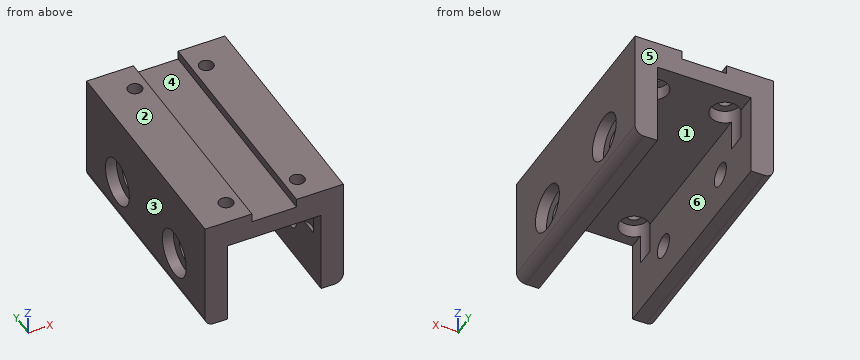
from build123d import *

# Parameters (mm, degrees)
PAD031_DEPTH            = 13.5
PAD031_DEPTH_BACK       = 38.5
SKETCH097_R             = 1.6
POCKET050_DEPTH         = 6.201
POCKET050_DEPTH_BACK    = 19.001
SKETCH100_R             = 3.25
POCKET051_DEPTH         = 10
LINEARPATTERN_COUNT     = 2
LINEARPATTERN_PITCH     = 25
BODY029_PLACEMENT_ANGLE = 180


with BuildPart() as part:
    # Sketch099 → Pad031 (new body, two sides)
    with BuildSketch(Plane.XZ) as pad031_sk:
        with BuildLine():
            Line((-13.5, 19), (-10.5, 19))
            Line((-10.5, 0), (-10.5, 19))
            Line((10.5, 0), (-10.5, 0))
            Line((10.5, 19), (10.5, 0))
            Line((10.5, 19), (13.5, 19))
            ThreePointArc((15.5, 17), (14.914214, 18.414214), (13.5, 19))
            Line((15.5, 17), (15.5, -6.2))
            Line((15.5, -6.2), (5, -6.2))
            Line((5, -4.2), (5, -6.2))
            Line((-5, -4.2), (5, -4.2))
            Line((-5, -6.2), (-5, -4.2))
            Line((-5, -6.2), (-15.5, -6.2))
            Line((-15.5, -6.2), (-15.5, 17))
            ThreePointArc((-13.5, 19), (-14.914214, 18.414214), (-15.5, 17))
        make_face()
    extrude(amount=PAD031_DEPTH)
    extrude(pad031_sk.sketch, amount=-PAD031_DEPTH_BACK)

    # Sketch097 → Pocket050 (cut, two sides)
    with BuildSketch(Plane.XY) as pocket050_sk:
        with Locations((-8, 32)):
            Circle(SKETCH097_R)
        with Locations((8, 32)):
            Circle(SKETCH097_R)
        with Locations((-8, -8)):
            Circle(SKETCH097_R)
        with Locations((8, -8)):
            Circle(SKETCH097_R)
    extrude(amount=-POCKET050_DEPTH, mode=Mode.SUBTRACT)
    extrude(pocket050_sk.sketch, amount=POCKET050_DEPTH_BACK, mode=Mode.SUBTRACT)

    # Sketch100 → Pocket051 (cut)
    with BuildSketch(Plane(origin=(0, 0, -3), x_dir=(-1, 0, 0), z_dir=(0, 0, -1))):
        with Locations((-8, 32)):
            Circle(SKETCH100_R)
        with Locations((8, 32)):
            Circle(SKETCH100_R)
        with Locations((-8, -8)):
            Circle(SKETCH100_R)
        with Locations((8, -8)):
            Circle(SKETCH100_R)
    extrude(amount=-POCKET051_DEPTH, mode=Mode.SUBTRACT)

    # Sketch110 → Groove (revolve, cut)
    with BuildSketch(Plane(origin=(0, 0, 10), x_dir=(-1, 0, 0), z_dir=(0, 1, 0))):
        Polygon((-13, 2.65), (13, 2.65), (13, 5.25), (23, 5.25), (23, 0), (-23, 0), (-23, 5.25), (-13, 5.25), align=None)
    groove = revolve(axis=Axis((0, 0, 10), (-1, 0, 0)), mode=Mode.SUBTRACT)

    # LinearPattern: Groove ×2
    with Locations(*[(0, i * LINEARPATTERN_PITCH, 0) for i in range(1, LINEARPATTERN_COUNT)]):
        add(groove, mode=Mode.SUBTRACT)


with BuildPart() as part_1:
    # Body029 placement: moved
    add(part.part.moved(Location((0, 0, 32))).rotate(Axis((0, 0, 32), (0, 1, 0)), BODY029_PLACEMENT_ANGLE))


solid = part_1.part
Geometry: final body of the model. Coordinates: model frame, mm. Face numbers are marked on the shaded views. A direction names the side the tool comes from. Give positions to 0.01 mm unless a question says otherwise; leave off trailing zeros. Order: outer loops, then holes, each group sorted by start corner. A loop starts at its lowest first (then second) coordinate and runs counter-clockwise, first axis right, second up. Notation, with made-up numbers: (71, 43) -> (129, 43) arc R17 cw to (129, 59) -> close; hole circle Ø5 at (86, -34.5). An arc over 180 degrees is marked (long way). Put each result on its own line as item: value.
Q1. Reachability of the marked faces 1 and 2 from +Z, -Z, +X, -X, +Y, -Y: full face, straight path, thin tool, end or side. Return the list, or none.
Here are the results:
face 1: -Z, +Y, -Y
face 2: +Z, +X, -X, +Y, -Y
Q2. Pin query (flat end, axial travel): pin 1 (2.5 mm diameter, centred on x = 8, y = 32, fed in from +Z); pin 2 (7 mm diameter, centred on y = 25, z = 22, fed in from -X); pin 3 (10.5 mm diameter, centred on x = -8, y = -8, fed in from +Z); pin 4 (6 mm diameter, centred on x = 5.5, y = 24.5, fed in from -Z). Return the tip coordinate at first contact, or that it passes through.
Here are the results:
pin 1: passes through
pin 2: stops at x = -13
pin 3: stops at z = 38.2
pin 4: stops at z = 32
Q3. Section A-A, the plane y = -8. Count the separate pieces of the cut face and the enclosed holes in it, then the cut area to 3 significant figures.
Here are the results:
separate pieces: 3
enclosed holes: 0
area: 291 mm^2
Q4. Draft query along X for the marked faces 3, 4, 5 and 6. Return one class per face: released by +X, released by -X, zero draft, split by the parting line, or undercut.
Here are the results:
face 3: released by -X
face 4: undercut
face 5: zero draft
face 6: undercut
Q5. Section B-B, the plane x = -8. Return loops of the section in (y, z).
Here are the results:
outline: (-13.5, 32) -> (-11.25, 32) -> (-11.25, 35) -> (-9.6, 35) -> (-9.6, 38.2) -> (-13.5, 38.2) -> close; (-6.4, 35) -> (-4.75, 35) -> (-4.75, 32) -> (28.75, 32) -> (28.75, 35) -> (30.4, 35) -> (30.4, 38.2) -> (-6.4, 38.2) -> close; (33.6, 35) -> (35.25, 35) -> (35.25, 32) -> (38.5, 32) -> (38.5, 38.2) -> (33.6, 38.2) -> close
Q6. Section C-C, the plane z = 33. Return loops of the section in (x, y).
Here are the results:
outline: (-15.5, -13.5) -> (15.5, -13.5) -> (15.5, 38.5) -> (-15.5, 38.5) -> close; hole circle Ø6.5 at (-8, -8); hole circle Ø6.5 at (-8, 32); hole circle Ø6.5 at (8, -8); hole circle Ø6.5 at (8, 32)
Q7. Material intervals for L1, parallel to Y at x = -11.4, z = 22; L2, parallel to X at y = 18, z = 21.25; L3, parallel to X at y = 12, z = 36.75, sorted ascending.
Here are the results:
L1: y = -13.5 to -2.65, 2.65 to 22.35, 27.65 to 38.5
L2: x = -15.5 to -10.5, 10.5 to 15.5
L3: x = -15.5 to -5, 5 to 15.5
